```python
from build123d import *

# Parameters (mm, degrees)
SKETCH1_W           = 55
SKETCH1_H           = 30
BOSS_EXTRUDE1_DEPTH = 30
SKETCH2_W           = 13
SKETCH2_H           = 56
BOSS_EXTRUDE2_DEPTH = 35
SKETCH3_W           = 5.5
SKETCH3_H           = 11
CUT_EXTRUDE1_DEPTH  = 22


with BuildPart() as part:
    # Sketch1 → Boss-Extrude1 (new body)
    with BuildSketch(Plane(origin=(0, 0, 0), x_dir=(1, 0, 0), z_dir=(0, 1, 0))):
        Rectangle(SKETCH1_W, SKETCH1_H)
    extrude(amount=BOSS_EXTRUDE1_DEPTH)

    # Sketch2 → Boss-Extrude2 (add)
    with BuildSketch(Plane.XY.offset(15)):
        with Locations((1, 28)):
            Rectangle(SKETCH2_W, SKETCH2_H)
    extrude(amount=BOSS_EXTRUDE2_DEPTH)

    # Sketch3 → Cut-Extrude1 (cut)
    with BuildSketch(Plane.XY.offset(50)):
        with Locations((1, 20.5)):
            Rectangle(SKETCH3_W, SKETCH3_H)
        with Locations((1, 47.5)):
            Rectangle(SKETCH3_W, SKETCH3_H)
    extrude(amount=-CUT_EXTRUDE1_DEPTH, mode=Mode.SUBTRACT)


solid = part.part
```
Read the model definition and answer for the solid it produces. Units are mm, in the model's axes. A direction names the side the tool comes from. Give positions to 0.01 mm unless a question says otherwise; leave off trailing zeros. Order: outer loops, then holes, each group sorted by start corner. A loop starts at its lowest first (then second) coordinate and runs counter-clockwise, first axis right, second up. Notation, with made-up numbers: (87, 22.25) -> (103, 22.25) arc R23 ccw to (103, 38.25) -> close; hole circle Ø4 at (13, 84). An arc over 180 degrees is marked (long way). Write item = value, one per line.
1. The mould has two halves that part along X. Classify faces 1 (the face through (17, 15, 15)), 2 (the face through (-27.5, 15, 0)), 3 (the face through (1, 42, 39)): +X half, -X half, draft (parallel to the pull), parting line (faces both ways), or undercut.
Numbers:
face_1 = draft
face_2 = -X half
face_3 = undercut
2. Straight lines are drawn through the part: line 1 along X through (y, z) = (21, 33.5); line 2 along Y through (x, z) = (1, 40); line 3 along Z through (x, y) = (19, 5.5). For each, find the intervals that lie inside material, in ascending order.
Numbers:
line_1 = -5.5 to -1.75, 3.75 to 7.5
line_2 = 0 to 15, 26 to 42, 53 to 56
line_3 = -15 to 15
3. Given pin 1 (12 mm diameter, centred on y = 21, z = 34, fed in from +X); pin 2 (8 mm diameter, centred on x = -9.5, z = 14, fed in from +Y); pin 3 (3 mm diameter, centred on x = -17, y = 28.5, fed in from +Z), each flat-ended and moving along its own axis, determine where each tip first touches the part or whether it passes through.
Numbers:
pin_1 = 7.5
pin_2 = 30
pin_3 = 15
4. A cutting plane is placed at C-C, the plane y = 48.5. Write down the section's boundary in (x, z), and give its area (3 significant figures).
Numbers:
outline = (-5.5, 15) -> (7.5, 15) -> (7.5, 50) -> (3.75, 50) -> (3.75, 28) -> (-1.75, 28) -> (-1.75, 50) -> (-5.5, 50) -> close
area = 334 mm²
5. For faces 4 (the face through (1, 43, 15)), 5 (the face through (1, 15, 39)), 6 (the face through (7.5, 28, 32)), 7 (the face through (-17, 15, 15)), determine the directions among +Z, -Z, +X, -X, +Y, -Y from which every point of the face is accessible in a straight line to the end or side of a thin tool.
Numbers:
face_4 = -Z, +X, -X, +Y
face_5 = +Z
face_6 = +Z, +X, +Y, -Y
face_7 = +Z, -X, +Y, -Y
6. A cutting plane is placed at D-D, the plane z = 17. Write down the section's boundary in (x, y), and give its area (3 significant figures).
Numbers:
outline = (-5.5, 0) -> (7.5, 0) -> (7.5, 56) -> (-5.5, 56) -> close
area = 728 mm²
7. A cutting plane is placed at B-B, the plane x = 0. Write down the section's boundary in (y, z).
Numbers:
outline = (0, -15) -> (30, -15) -> (30, 15) -> (56, 15) -> (56, 50) -> (53, 50) -> (53, 28) -> (42, 28) -> (42, 50) -> (26, 50) -> (26, 28) -> (15, 28) -> (15, 50) -> (0, 50) -> close
8. A cutting plane is placed at A-A, the plane z = 46. Write down the section's boundary in (x, y).
Numbers:
outline = (-5.5, 0) -> (7.5, 0) -> (7.5, 56) -> (-5.5, 56) -> close; hole (-1.75, 15) -> (3.75, 15) -> (3.75, 26) -> (-1.75, 26) -> close; hole (-1.75, 42) -> (3.75, 42) -> (3.75, 53) -> (-1.75, 53) -> close
